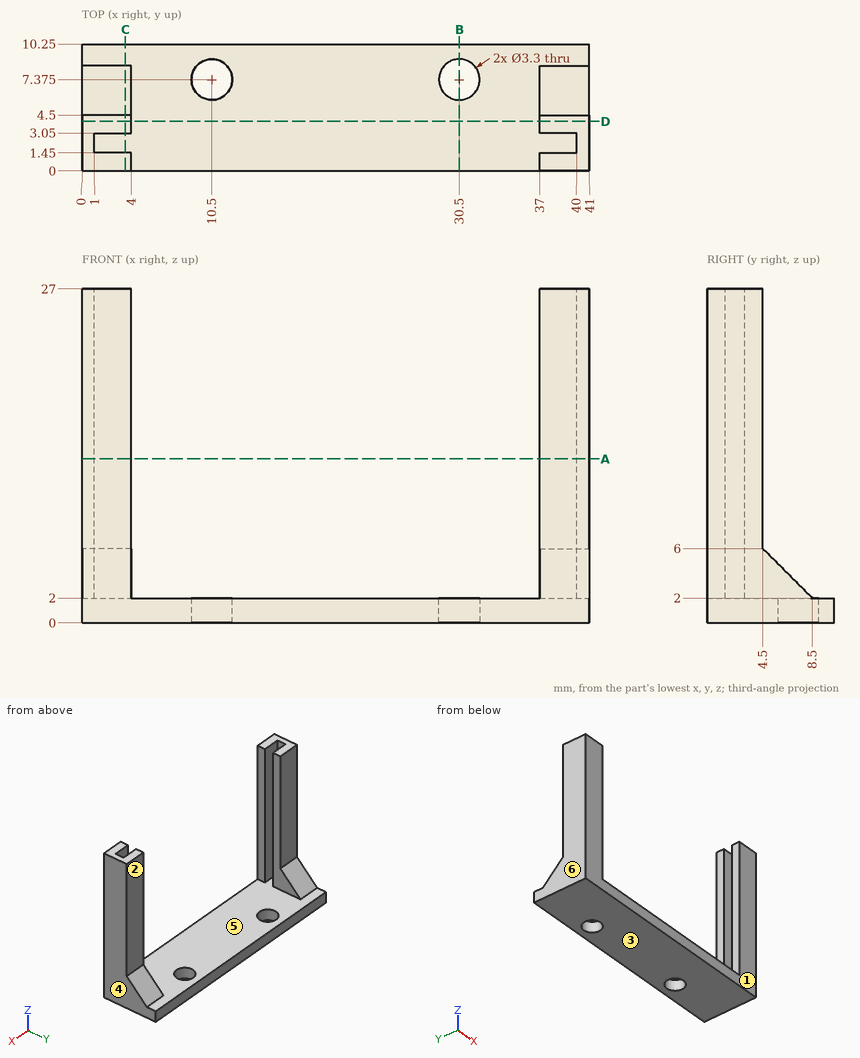
Here's the drawing with two shaded views (mm, measured from the low corner). I have some questions. A direction names the side the tool comes from. Give positions to 0.01 mm unless a question says otherwise; leave off trailing zeros. Loops run counter-clockwise (first coordinate to the right, second up) from the corner with the lowest first, then second, coordinate; pieces in that order, holes last. Notation, with made-up numbers: M 18.5,88.5 L 68.5,88.5 A22 ccw 68.5,115.5 Z; hole C 57.5,67.25 d1. An arc over 180 degrees is marked long. One line per item, written item: value.
1) On a 3-axis mill with a long thin cutter (end or side, diameter ignored), from which of +Z, -Z, +X, -X, +Y, -Y can I reach the whole of each face in a straight line? I mean the marked faces 1 and 2. Say none if no direction works.
Geometry check:
face 1: +Z, -Z, +X, -X, -Y
face 2: +Z, +X, -X, +Y
2) Imagine slicing it at B-B on x = 30.5. Write out the boundary of the cut face in (y, z) (3 decimals).
Geometry check:
outline: M 0,0 L 5.725,0 L 5.725,2 L 0,2 Z; M 9.025,0 L 10.25,0 L 10.25,2 L 9.025,2 Z
3) Imagine slicing it at C-C on x = 3.5. Write out the boundary of the cut face in (y, z).
Geometry check:
outline: M 0,0 L 10.25,0 L 10.25,2 L 8.5,2 L 4.5,6 L 4.5,27 L 3.05,27 L 3.05,2 L 1.45,2 L 1.45,27 L 0,27 Z
4) I'm going to push flat-ended pins straight in: pin 1 (3.5 mm diameter, centred on x = 38, z = 9, fed in from +Y); pin 2 (5 mm diameter, centred on x = 22, y = 4.5, fed in from +Z). Where does each tip first touch, or does it pass through?
Geometry check:
pin 1: stops at y = 4.5
pin 2: stops at z = 2
5) Thinking about a two-plate mould opening in X: for the marked faces 3, 4, 5 and 6, which applies, +X half, -X half, draft (parallel to the pull), parting line (faces both ways), or undercut?
Geometry check:
face 3: draft
face 4: +X half
face 5: undercut
face 6: -X half
6) Imagine slicing it at A-A on z = 13.25. Write out the boundary of the cut face in (x, y), and give its area (3 significant figures).
Geometry check:
outline: M 0,0 L 4,0 L 4,1.45 L 1,1.45 L 1,3.05 L 4,3.05 L 4,4.5 L 0,4.5 Z; M 37,0 L 41,0 L 41,4.5 L 37,4.5 L 37,3.05 L 40,3.05 L 40,1.45 L 37,1.45 Z
area: 26.4 mm²
7) Please list where these lines run through material, in increasing order: line 1 (X direction, y = 3.25, z = 23.5); line 2 (Y direction, x = 2.5, z = 13.25); line 3 (X direction, y = 2.25, z = 16.75).
Geometry check:
line 1: x = 0 to 4, 37 to 41
line 2: y = 0 to 1.45, 3.05 to 4.5
line 3: x = 0 to 1, 40 to 41
8) Imagine slicing it at D-D on y = 4. Write out the boundary of the cut face in (x, z).
Geometry check:
outline: M 0,0 L 41,0 L 41,27 L 37,27 L 37,2 L 4,2 L 4,27 L 0,27 Z
